```python
from build123d import *

# Parameters (mm, degrees)
SKETCH015_W     = 10.932014
SKETCH015_H     = 6.638581
PAD007_DEPTH    = 0.4
SKETCH016_W     = 3.5
SKETCH016_H     = 3.5
PAD008_DEPTH    = 4
SKETCH017_W     = 2
SKETCH017_H     = 2
POCKET008_DEPTH = 3


with BuildPart() as part:
    # Sketch015 → Pad007 (new body)
    with BuildSketch(Plane.XY.offset(13)):
        with Locations((9.503802, 14.425956)):
            Rectangle(SKETCH015_W, SKETCH015_H)
    extrude(amount=PAD007_DEPTH)

    # Sketch016 (on Face6 of Pad007) → Pad008 (join)
    with BuildSketch(Plane.XY.offset(13.4)):
        with Locations((10.165375, 14.45904)):
            Rectangle(SKETCH016_W, SKETCH016_H)
    extrude(amount=PAD008_DEPTH)

    # Sketch017 (on Face4 of Pad008) → Pocket008 (cut)
    with BuildSketch(Plane(origin=(0, 0, 13), x_dir=(1, 0, 0), z_dir=(0, 0, -1))):
        with Locations((10.13506, -14.402274)):
            Rectangle(SKETCH017_W, SKETCH017_H)
    extrude(amount=-POCKET008_DEPTH, mode=Mode.SUBTRACT)


with BuildPart() as part_1:
    # Body006 placement: moved
    add(part.part.moved(Location((0, 0, -4))))


solid = part_1.part
```
Work out the finished part from the listing and answer in its coordinate system (mm). A direction names the side the tool comes from. Coordinates: 2 decimals unless noted, no trailing zeros. Write each loop counter-clockwise with the first axis right and the second up, starting at its lowest first coordinate (ties: lowest second). Pieces come first, ordered by that corner, then holes.
Q1. A cutting plane is placed at B-B, the plane y = 14.5. Give the vertices of the cut face in (x, z), then the cut area to 3 significant figures.
Q2. Which of the six approach directions +Z, -Z, +X, -X, +Y, -Y give full straight-line access (tool end or side, diameter ignored) to faces 1 (the face through (10, 12.709, 11)), 2 (the face through (8.415, 14, 11)), 3 (the face through (10, 16.209, 11)), 4 (the face through (10, 14, 13.4)), 5 (the face through (10, 14, 12))?
Q3. A cutting plane is placed at A-A, the plane z = 11.4. Give the vertices of the cut face in (x, y).
Q4. Find the intervals of material crossed by line 1 (Y direction, x = 9.25, z = 10.2); line 2 (X direction, y = 14, z = 11.55); line 3 (Z direction, x = 12.75, y = 11.5), in increasing order.
Q5. Determine the mould class of faces 6 (the face through (11.915, 14, 11)), 7 (the face through (9.135, 14, 10)), 8 (the face through (8, 14, 9.4)), 9 (the face through (10, 15.402, 10)) for opening direction X: released by +X, released by -X, zero draft, split by the parting line, or undercut.
Q6. A cutting plane is placed at C-C, the plane x = 11. Give the vertices of the cut face in (y, z), then the cut area to 3 significant figures.
Q7. Each of these flat-tipped pins is pushed along its axis until it touches: pin 1 Ø1.8 at (x, z) = (10.5, 11) entering from +Y; pin 2 Ø1 at (y, z) = (13, 12) entering from +X; pin 3 Ø1 at (y, z) = (14.5, 10.5) entering from -X; pin 4 Ø2 at (x, y) = (10.5, 14.5) entering from -Z. Where does it stop, or does it pass through?
Q8. A cutting plane is placed at D-D, the plane z = 13. Give the vertices of the cut face in (x, y).
Findings below:
1. outline: (4.04, 9) - (9.14, 9) - (9.14, 12) - (11.14, 12) - (11.14, 9) - (14.97, 9) - (14.97, 9.4) - (11.92, 9.4) - (11.92, 13.4) - (8.42, 13.4) - (8.42, 9.4) - (4.04, 9.4) - close
1. area: 12.4 mm2
2. face 1: +Z, +X, -X, -Y
2. face 2: +Z, -X, +Y, -Y
2. face 3: +Z, +X, -X, +Y
2. face 4: +Z, +X, -X, +Y, -Y
2. face 5: -Z
3. outline: (8.42, 12.71) - (11.92, 12.71) - (11.92, 16.21) - (8.42, 16.21) - close; hole (9.14, 13.4) - (11.14, 13.4) - (11.14, 15.4) - (9.14, 15.4) - close
4. line 1: y = 12.71 to 13.4, 15.4 to 16.21
4. line 2: x = 8.42 to 9.14, 11.14 to 11.92
4. line 3: z = 9 to 9.4
5. face 6: released by +X
5. face 7: undercut
5. face 8: zero draft
5. face 9: undercut
6. outline: (11.11, 9) - (13.4, 9) - (13.4, 12) - (15.4, 12) - (15.4, 9) - (17.75, 9) - (17.75, 9.4) - (16.21, 9.4) - (16.21, 13.4) - (12.71, 13.4) - (12.71, 9.4) - (11.11, 9.4) - close
6. area: 10.7 mm2
7. pin 1: stops at y = 16.21
7. pin 2: stops at x = 11.92
7. pin 3: stops at x = 8.42
7. pin 4: stops at z = 9
8. outline: (8.42, 12.71) - (11.92, 12.71) - (11.92, 16.21) - (8.42, 16.21) - close
